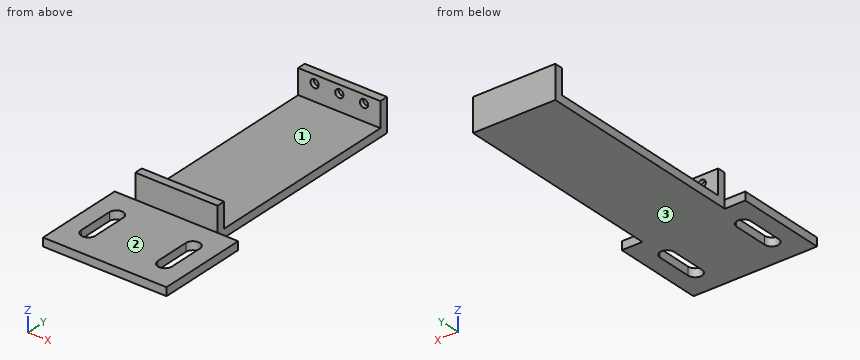
Solid Edge part; units mm, degrees
sketch "Sketch1" plane through (0, 0, 0) normal (0, 0, 1) x (1, 0, 0)
  line L0 (100, 0) -> (100, 260)
  line L1 (100, 260) -> (0, 260)
  line L2 (0, 260) -> (0, 0)
  line L3 (0, 0) -> (100, 0)
extrude "Protrusion1" add sketch "Sketch1" along normal blind 10
sketch "Sketch2" plane through (50, 130, 10) normal (0, 0, 1) x (1, 0, 0)
  line L0 (-50, 130) -> (50, 130)
  line L1 (50, 130) -> (50, 120)
  line L2 (50, 120) -> (-50, 120)
  line L3 (-50, 120) -> (-50, 130)
  line L4 (-50, -120) -> (50, -120)
  line L5 (50, -120) -> (50, -130)
  line L6 (50, -130) -> (-50, -130)
  line L7 (-50, -130) -> (-50, -120)
extrude "ExtrudedCutout_1" add sketch "Sketch2" along normal blind 30
hole "Hole_1" at (20, 250, 30) direction (0, 1, 0) diameter 10 depth 5
hole "Hole1" at (50, 250, 30) direction (0, 1, 0) diameter 10 depth 5
hole "Hole2" at (80, 250, 30) direction (0, 1, 0) diameter 10 depth 5
hole "Hole_4" at (80, 10, 30) direction (0, -1, 0) diameter 10 depth 5
hole "Hole3" at (50, 10, 30) direction (0, -1, 0) diameter 10 depth 5
hole "Hole4" at (20, 10, 30) direction (0, -1, 0) diameter 10 depth 5
sketch "Sketch3" plane through (50, 0, 15) normal (0, -1, 0) x (0, 0, 1)
  line L0 (-5, -75) -> (-15, -75)
  line L1 (-15, -75) -> (-15, 75)
  line L2 (-15, 75) -> (-5, 75)
  line L3 (-5, 75) -> (-5, -75)
extrude "ExtrudedProtrusion_5" add sketch "Sketch3" along normal blind 110
sketch "Sketch4" plane through (50, -55, 10) normal (0, 0, 1) x (-1, 0, 0)
  arc A0 (-55, 21.5) -> (-38, 21.5) centre (-46.5, 21.5) cw
  line L0 (-55, -21.5) -> (-55, 21.5)
  arc A1 (-38, -21.5) -> (-55, -21.5) centre (-46.5, -21.5) cw
  line L1 (-38, -21.5) -> (-38, 21.5)
  arc A2 (38, 21.5) -> (55, 21.5) centre (46.5, 21.5) cw
  line L2 (38, -21.5) -> (38, 21.5)
  arc A3 (55, -21.5) -> (38, -21.5) centre (46.5, -21.5) cw
  line L3 (55, -21.5) -> (55, 21.5)
extrude "Cutout1" cut sketch "Sketch4" against normal up to next
CAD build for the part. Positions are in the model's coordinates, mm. Face numbers are marked on the shaded views. A direction names the side the tool comes from. Round coordinates to 2 decimals unless told otherwise and drop trailing zeros. Loops run counter-clockwise (first coordinate to the right, second up) from the corner with the lowest first, then second, coordinate; pieces in that order, holes last. Notation, with made-up numbers: M 34.5,73 L 75.5,73 A9 ccw 75.5,87 Z; hole C 88.5,6 d11. An arc over 180 degrees is marked long. Use a Markdown table: item, result. Add a question column.
(1) Cut at B-B (x = 96.5). Give the cut face in (y, z).
(2) Cut at A-A (z = 16). Give the cut face in (x, y).
(3) Drill centre lines: line 1 (X direction, y = 7.5, z = 30); line 2 (Y direction, x = 21, z = 31); line 3 (Z direction, x = 20, y = 7.15). Where is each one in solid material? Low to high.
(4) Cut at C-C (x = 20). Give the cut face in (y, z), and give its area (3 significant figures).
(5) Which spindle directions (+Z, -Z, +X, -X, +Y, -Y) get a long thin tool onto all of the face, cutting with end or side? Do the marked faces 1, 2 and 3. Say none if no direction does.
(6) Cut at D-D (y = 70). Give the cut face in (x, z).
(7) Flat gauge pins, fed straight in: pin 1 (4 mm diameter, centred on x = 109, z = 5.5, fed in from +Y); pin 2 (12 mm diameter, centred on x = 79.5, z = 18, fed in from -Y); pin 3 (1 mm diameter, centred on y = 80.5, z = 8.5, fed in from +X); pin 4 (10 mm diameter, centred on x = 5.5, y = -47.5, fed in from +Z). Where does each tip first touch, or does it go through?
Geometry says:
| question | item | result |
|---|---|---|
| 1 | outline | M -110,0 L -85,0 L -85,10 L -110,10 Z; M -25,0 L 260,0 L 260,40 L 250,40 L 250,10 L 10,10 L 10,40 L 0,40 L 0,10 L -25,10 Z |
| 2 | outline | M 0,0 L 100,0 L 100,10 L 0,10 Z; M 0,250 L 100,250 L 100,260 L 0,260 Z |
| 3 | line 1 | x = 0 to 15, 25 to 45, 55 to 75, 85 to 100 |
| 3 | line 2 | y = 0 to 5, 255 to 260 |
| 3 | line 3 | z = 0 to 25, 35 to 40 |
| 4 | outline | M -110,0 L 260,0 L 260,40 L 250,40 L 250,35 L 255,35 L 255,25 L 250,25 L 250,10 L 10,10 L 10,25 L 5,25 L 5,35 L 10,35 L 10,40 L 0,40 L 0,10 L -110,10 Z |
| 4 | area | 4,200 mm² |
| 5 | face 1 | +Z, +X, -X |
| 5 | face 2 | +Z, +X, -X, -Y |
| 5 | face 3 | -Z, +X, -X, +Y, -Y |
| 6 | outline | M 0,0 L 100,0 L 100,10 L 0,10 Z |
| 7 | pin 1 | stops at y = 0 |
| 7 | pin 2 | stops at y = 0 |
| 7 | pin 3 | stops at x = 100 |
| 7 | pin 4 | passes through |
